Read the model definition and answer for the solid it produces. Units are mm, in the model's axes. A direction names the side the tool comes from. Give positions to 0.01 mm unless a question says otherwise; leave off trailing zeros. Loops run counter-clockwise (first coordinate to the right, second up) from the corner with the lowest first, then second, coordinate; pieces in that order, holes last. Notation, with made-up numbers: (13, -21) - (26, -21) arc R9 ccw to (26, -8) - close; hole circle Ø6 at (2, 47.25). An arc over 180 degrees is marked (long way). Write each question's results on one line, items separated by ' | '. Start each with the question number.
Q1. Given pin 1 (10 mm diameter, centred on x = -3.5, z = 27.5, fed in from -Y); pin 2 (17.5 mm diameter, centred on x = -60, y = -14.25, fed in from -Z); pin 3 (1 mm diameter, centred on y = -14, z = 22.5, fed in from +X); pin 4 (6 mm diameter, centred on y = 6, z = 18.5, fed in from -X), each flat-ended and moving along its own axis, determine where each tip first touches the part or whether it passes through.
Q2. For faces 1 (the flat face through (-11, 6, 25)), 2 (the flat face through (1, -26, 9)), 3 (the flat face through (17, -10, 25)), 4 (the flat face through (-30, 16, 25)), determine the directions among +Z, -Z, +X, -X, +Y, -Y from which every point of the face is accessible in a straight line to the end or side of a thin tool.
Q3. The part is cut by section D-D, the plane x = 13. Write down the section's boundary in (y, z).
Q4. The part is cut by section C-C, the plane y = -6. Write down the section's boundary in (x, z).
Q5. The part is cut by section B-B, the plane z = 4. Write down the section's boundary in (x, y).
Q6. The part is cut by section A-A, the plane x = 60. Write down the section's boundary in (y, z), plus the area to 3 significant figures.
Q7. Determine the mould class of faces 5 (the flat face through (24, 6, 25)), 6 (the flat face through (30, 16, 25)), 7 (the cylindrical face through (-64.638, -17.207, 7.395)) for opening direction X: +X half, -X half, draft (parallel to the pull), parting line (faces both ways), or undercut.
Q8. Find the intervals of material crossed by line 1 (X direction, y = -14.25, z = 5); line 2 (X direction, y = -19, z = 6.5); line 3 (Y direction, x = -60, z = 4.25), in increasing order. Write a range as from..to.
Autodesk Inventor part; units mm, degrees
ref_plane "Work Plane1" through (-30, 6, 35) normal (0, -0.8660254, -0.5) x (1, 0, 0)
ref_plane "YZ Plane" through (0, 0, 0) normal (1, 0, 0) x (0, 1, 0)
ref_plane "XZ Plane" through (0, 0, 0) normal (0, 1, 0) x (-1, 0, 0)
sketch "Sketch1" plane through (0, 0, 0) normal (0, 0, 1) x (1, 0, 0)
  line L0 (-68, 26) -> (68, 26)
  line L1 (68, 26) -> (68, -26)
  line L2 (68, -26) -> (-68, -26)
  line L3 (-68, -26) -> (-68, 26)
  point P0 (0, 0)
  point P1 (-68, 0)
  point P2 (0, 26)
  dimension "d0" = 136
  dimension "d1" = 52
extrude "Extrusion1" add sketch "Sketch1" along normal blind 15
sketch "Sketch9" plane through (0, 0, 15) normal (0, 0, 1) x (1, 0, 0)
  circle A0 centre (-60, -14.25) radius 4
  line L0 (188.1551, -73.0673) -> (-511.8449, -73.0673)
  circle A1 centre (60, -14.25) radius 4
  point P0 (0, 0)
hole "Hole3" at (-60, -14.25, 15) at (60, -14.25, 15) direction (0, 0, -1) diameter 11 end through all
sketch "Sketch10" plane through (0, 0, 15) normal (0, 0, 1) x (1, 0, 0)
  line L0 (30, 6) -> (-30, 6)
  line L1 (-30, 6) -> (-30, 26)
  line L2 (-30, 26) -> (30, 26)
  line L3 (30, 26) -> (30, 6)
  line L4 (-68, -26) -> (68, -26)
  line L5 (68, 26) -> (-68, 26)
  point P0 (0, 0)
  point P1 (0, 6)
  dimension "d47" = 60
  dimension "d56" = 20
extrude "Extrusion6" add sketch "Sketch10" along normal blind 20
ref_plane "Work Plane1" through (-30, 6, 35) normal (0, -0.8660254, -0.5) x (1, 0, 0)
sketch "Sketch11" plane through (-30, 6, 35) normal (0, -0.8660254, -0.5) x (1, 0, 0)
  circle A0 centre (30, -10) radius 5
  line L0 (0, 0) -> (60, 0)
  point P0 (30, -27.3109)
  point P1 (30, 0)
  dimension "d52" = 10
  dimension "d53" = 10
extrude "Extrusion7" cut sketch "Sketch11" against normal blind 33
sketch "Sketch12" plane through (0, 11, 26.3397) normal (0, 0.8660254, 0.5) x (1, 0, 0)
  circle A0 centre (0, 0) radius 5
  point P0 (0, 17.3109)
extrude "Extrusion8" cut sketch "Sketch12" against normal up to surface surface through (-30, 6, 15) normal (0, -1, 0)
sketch "Sketch13" plane through (0, 0, 15) normal (0, 0, 1) x (1, 0, 0)
  line L0 (17, -26) -> (7, -26)
  line L1 (7, -26) -> (7, 6)
  line L2 (7, 6) -> (17, 6)
  line L3 (17, 6) -> (17, -26)
  line L4 (-30, 6) -> (30, 6)
  line L5 (-68, -26) -> (68, -26)
  ellipse E0 centre (0, 26) end of major axis (0, 36) minor radius 5 (-5, 26) -> (5, 26) ccw
  line L6 (5, 6) -> (-5, 6)
  point P0 (0, 0)
  dimension "d59" = 10
  dimension "d62" = 2
extrude "Extrusion9" add sketch "Sketch13" along normal up to surface (20 mm away)
sketch "Sketch14" plane through (7, -26, 15) normal (-1, 0, 0) x (0, 0, 1)
  line L0 (0, 0) -> (20, 0)
  point P0 (-15, 26)
  point P1 (10, 10)
  point P2 (10, 20)
  point P3 (10, 0)
  dimension "d65" = 10
  dimension "d66" = 10
hole "Hole4" at (7, -16, 25) at (7, -6, 25) direction (1, 0, 0) diameter 5 end through all
properties part number "0008-30-014"
Check sheet entries:
1) pin 1: stops at y = 6 | pin 2: stops at z = 0 | pin 3: stops at x = 17 | pin 4: stops at x = -30
2) face 1: +Z, -X, -Y | face 2: +Z, -Z, +X, -X, -Y | face 3: +Z, +X, -Y | face 4: +Z, -X, +Y, -Y
3) outline: (-26, 0) - (26, 0) - (26, 35) - (-26, 35) - close; hole circle Ø5 at (-16, 25); hole circle Ø5 at (-6, 25)
4) outline: (-68, 0) - (68, 0) - (68, 15) - (17, 15) - (17, 22.5) - (7, 22.5) - (7, 15) - (-68, 15) - close; (7, 27.5) - (17, 27.5) - (17, 35) - (7, 35) - close
5) outline: (-68, -26) - (68, -26) - (68, 26) - (-68, 26) - close; hole circle Ø11 at (-60, -14.25); hole circle Ø11 at (60, -14.25)
6) outline: (-26, 0) - (-19.75, 0) - (-19.75, 15) - (-26, 15) - close; (-8.75, 0) - (26, 0) - (26, 15) - (-8.75, 15) - close | area: 615 mm^2
7) face 5: draft | face 6: +X half | face 7: undercut
8) line 1: x = -68..-65.5, -54.5..54.5, 65.5..68 | line 2: x = -68..-62.77, -57.23..57.23, 62.77..68 | line 3: y = -26..-19.75, -8.75..26
